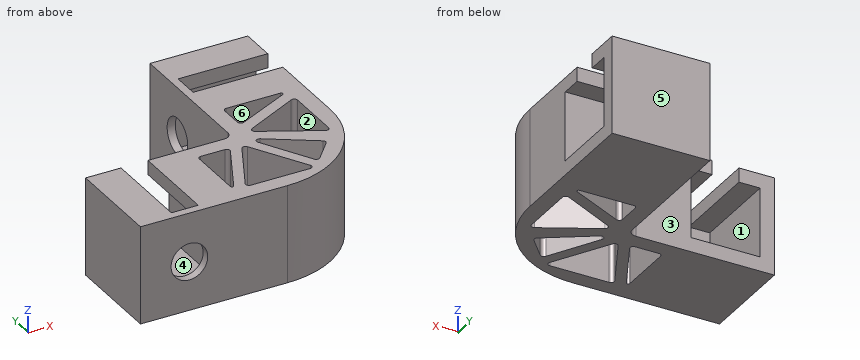
Autodesk Inventor part; units mm, degrees
ref_plane "YZ Plane" through (0, 0, 0) normal (1, 0, 0) x (0, 1, 0)
ref_plane "XZ Plane" through (0, 0, 0) normal (0, 1, 0) x (-1, 0, 0)
ref_plane "XY Plane" through (0, 0, 0) normal (0, 0, 1) x (1, 0, 0)
sketch "Sketch1" plane through (0, 0, 0) normal (0, 0, 1) x (1, 0, 0)
  line L0 (0, 0) -> (150, 0)
  line L1 (150, 0) -> (150, 45)
  line L2 (90, 60) -> (0, 60)
  line L3 (0, 60) -> (0, 0)
  line L4 (90, 60) -> (90, 150)
  line L5 (90, 150) -> (150, 150)
  line L6 (150, 150) -> (150, 45)
  dimension "d5" = 90
  dimension "d6" = 60
  dimension "d7" = 90
  dimension "d9" = 60
  dimension "d10" = 150
  dimension "d11" = 150
extrude "Extrusion1" add sketch "Sketch1" along normal blind 60
sketch "Sketch2" plane through (0, 60, 0) normal (0, 1, 0) x (1, 0, 0)
  line L0 (0, 0) -> (150, 0) construction
  line L1 (0, 0) -> (60, -60) construction
  line L2 (0, 0) -> (84.8528, 0) construction
  line L3 (8.75, -51.25) -> (8.75, -8.75)
  line L4 (8.75, -8.75) -> (51.25, -8.75)
  line L5 (51.25, -8.75) -> (51.25, -51.25)
  line L6 (51.25, -51.25) -> (8.75, -8.75) construction
  line L7 (8.75, -51.25) -> (51.25, -8.75) construction
  line L8 (30, -30) -> (30, -51.25) construction
  line L9 (30, -51.25) -> (21.75, -51.25) construction
  line L10 (30, -51.25) -> (38.25, -51.25) construction
  line L11 (21.75, -51.25) -> (21.75, -60)
  line L12 (0, -60) -> (150, -60)
  line L13 (38.25, -51.25) -> (38.25, -60)
  line L14 (21.75, -60) -> (38.25, -60)
  line L15 (51.25, -51.25) -> (38.25, -51.25)
  line L16 (21.75, -51.25) -> (8.75, -51.25)
  dimension "d14" = 84.8528
  dimension "d15" = 45
  dimension "d16" = 42.5
  dimension "d17" = 42.5
  dimension "d32" = 8.25
  dimension "d33" = 8.25
  dimension "d34" = 90
extrude "Extrusion2" cut sketch "Sketch2" against normal blind 55
sketch "Sketch4" plane through (150, 0, 0) normal (1, 0, 0) x (0, 0, -1)
  line L0 (0, 150) -> (0, 60) construction
  line L1 (0, 150) -> (-60, 90) construction
  line L2 (0, 150) -> (84.8528, 150) construction
  line L3 (-51.25, 98.75) -> (-8.75, 98.75)
  line L4 (-8.75, 98.75) -> (-8.75, 141.25)
  line L5 (-8.75, 141.25) -> (-51.25, 141.25)
  line L6 (-51.25, 98.75) -> (-8.75, 141.25) construction
  line L7 (-8.75, 98.75) -> (-51.25, 141.25) construction
  line L8 (-30, 120) -> (-60, 120) construction
  line L9 (-60, 120) -> (-60, 128.25)
  line L10 (-60, 0) -> (-60, 150)
  line L11 (-60, 128.25) -> (-51.25, 128.25)
  line L12 (-60, 120) -> (-60, 111.75)
  line L13 (-60, 111.75) -> (-51.25, 111.75)
  line L14 (-51.25, 141.25) -> (-51.25, 128.25)
  line L15 (-51.25, 111.75) -> (-51.25, 98.75)
  point P0 (0, 0)
  dimension "d26" = 84.8528
  dimension "d27" = 135
  dimension "d28" = 42.5
  dimension "d29" = 42.5
  dimension "d35" = 8.25
  dimension "d36" = 8.25
  dimension "d37" = 90
extrude "Extrusion4" cut sketch "Sketch4" against normal blind 55
hole "Hole2" at (30, 5, 30) direction (0, -1, 0) diameter 22.5 end through all
hole "Hole4" at (95, 120, 30) direction (-1, 0, 0) diameter 22.5 end through all
fillet "Fillet1" radius 5 1 edges at (90, 60, 30)
fillet "Fillet2" radius 60 1 edges at (150, 0, 30)
sketch "Sketch5" plane through (0, 0, 60) normal (0, 0, 1) x (1, 0, 0)
  line L0 (0, 0) -> (90, 0) construction
  line L1 (0, 0) -> (60, 0) construction
  line L2 (60, 0) -> (60, 60) construction
  line L3 (60, 60) -> (0, 60) construction
  line L4 (0, 60) -> (0, 0) construction
  line L5 (149.6513, 150.4559) -> (89.6513, 150.4559) construction
  line L6 (89.6513, 150.4559) -> (89.6513, 90.4559) construction
  line L7 (89.6513, 90.4559) -> (149.6513, 90.4559) construction
  line L8 (149.6513, 90.4559) -> (149.6513, 150.4559) construction
  line L9 (89.6513, 90.4559) -> (149.6513, 90.4559) construction
  line L10 (149.6513, 90.4559) -> (149.6513, 80.4559) construction
  line L11 (149.6513, 80.4559) -> (89.6513, 80.4559) construction
  line L12 (89.6513, 80.4559) -> (89.6513, 90.4559) construction
  line L13 (60, 60) -> (70, 60) construction
  line L14 (70, 60) -> (70, 0) construction
  line L15 (70, 0) -> (60, 0) construction
  line L16 (60, 0) -> (60, 60) construction
  line L17 (70, 60) -> (89.6513, 60) construction
  line L18 (89.6513, 60) -> (89.6513, 80.4559) construction
  line L19 (89.6513, 80.4559) -> (70, 80.4559) construction
  line L20 (70, 80.4559) -> (70, 60) construction
  line L21 (70, 60) -> (90, 60) construction
  line L22 (90, 60) -> (90, 50) construction
  line L23 (90, 50) -> (70, 50) construction
  line L24 (70, 50) -> (70, 60) construction
  line L25 (90, 50) -> (100, 50) construction
  line L26 (100, 50) -> (100, 60.8297) construction
  line L27 (100, 60.8297) -> (90, 60.8297) construction
  line L28 (90, 60.8297) -> (90, 50) construction
  line L29 (100, 60.8297) -> (89.6513, 60.8297) construction
  line L30 (89.6513, 60.8297) -> (89.6513, 80.4559) construction
  line L31 (89.6513, 80.4559) -> (100, 80.4559) construction
  line L32 (100, 80.4559) -> (100, 60.8297) construction
  line L33 (149.6513, 80.4559) -> (139.6513, 80.4559) construction
  line L34 (139.6513, 80.4559) -> (139.6513, 0.4559) construction
  line L35 (139.6513, 0.4559) -> (149.6513, 0.4559) construction
  line L36 (149.6513, 0.4559) -> (149.6513, 80.4559) construction
  line L37 (70, 0) -> (139.6513, 0) construction
  line L38 (139.6513, 0) -> (139.6513, 10) construction
  line L39 (139.6513, 10) -> (70, 10) construction
  line L40 (70, 10) -> (70, 0) construction
  arc A0 (90, 0) -> (150, 60) centre (90, 60) ccw construction
  line L41 (123.1662, 10) -> (113.1662, 10) construction
  line L42 (113.1662, 10) -> (113.1662, 20) construction
  line L43 (113.1662, 20) -> (123.1662, 20) construction
  line L44 (123.1662, 20) -> (123.1662, 10) construction
  line L45 (123.1662, 20) -> (133.1662, 20) construction
  line L46 (133.1662, 20) -> (133.1662, 30) construction
  line L47 (133.1662, 30) -> (123.1662, 30) construction
  line L48 (123.1662, 30) -> (123.1662, 20) construction
  line L49 (133.1662, 30) -> (143.1662, 30) construction
  line L50 (143.1662, 30) -> (143.1662, 40) construction
  line L51 (143.1662, 40) -> (133.1662, 40) construction
  line L52 (133.1662, 40) -> (133.1662, 30) construction
  line L53 (70, 10) -> (90, 50)
  line L54 (113.1662, 10) -> (90, 50)
  line L55 (70, 10) -> (113.1662, 10)
  line L56 (100, 60.8297) -> (139.6513, 40)
  line L57 (100, 60.8297) -> (139.6513, 80.4559)
  line L58 (139.6513, 40) -> (139.6513, 80.4559)
  line L59 (113.1662, 10) -> (139.6513, 40) construction
  line L60 (90, 50) -> (100, 60.8297) construction
  line L61 (95, 55.4149) -> (117.8355, 15.289)
  line L62 (95, 55.4149) -> (131.9763, 31.3064)
  line L63 (117.8355, 15.289) -> (131.9763, 31.3064)
  line L64 (90, 50) -> (83, 50) construction
  line L65 (83, 50) -> (63.0073, 10)
  line L66 (63.0073, 10) -> (63.0073, 50)
  line L67 (63.0073, 50) -> (83, 50)
  line L68 (100, 69.1023) -> (139.6513, 88.1548)
  line L69 (139.6513, 88.1548) -> (100, 88.1548)
  line L70 (100, 88.1548) -> (100, 69.1023)
  dimension "d76" = 60
  dimension "d77" = 60
  dimension "d78" = 60
  dimension "d79" = 60
  dimension "d80" = 60
  dimension "d81" = 10
  dimension "d82" = 10
  dimension "d83" = 60
  dimension "d84" = 10
  dimension "d85" = 10
  dimension "d86" = 10
  dimension "d87" = 80
  dimension "d88" = 10
  dimension "d89" = 10
  dimension "d90" = 10
  dimension "d91" = 10
  dimension "d92" = 10
  dimension "d93" = 10
  dimension "d94" = 10
  dimension "d97" = 7
extrude "Extrusion5" cut sketch "Sketch5" against normal blind 94
fillet "Fillet3" radius 2 13 edges at (113.1662, 10, 30) (131.9763, 31.3064, 30) (117.8355, 15.289, 30) (70, 10, 30) (63.0073, 50, 30) (83, 50, 30) (90, 50, 30) (95, 55.4149, 30) (100, 60.8297, 30) (100, 69.1023, 30) (100, 88.1548, 30) (139.6513, 80.4559, 30) (139.6513, 40, 30)
fillet "Fillet4" radius 1 2 edges at (63.0073, 10, 30) (139.6513, 88.1548, 30)
properties part number "OuterFrame"
The listing builds one solid part. Answer for the finished solid, in the listing's coordinates (mm). Face numbers are marked on the shaded views. A direction names the side the tool comes from. Give positions to 0.01 mm unless a question says otherwise; leave off trailing zeros. Order: outer loops, then holes, each group sorted by start corner. A loop starts at its lowest first (then second) coordinate and runs counter-clockwise, first axis right, second up. Notation, with made-up numbers: (-13.5, 34) -> (39.5, 34) arc R28 ccw to (39.5, 62) -> close; hole circle Ø11 at (83, 85). An arc over 180 degrees is marked (long way). Answer as CSV lines item,"result". Start each with the question number.
Q1. A cutting plane is placed at B-B (y = 120). Determine the outline of the cut face in (x, z).
Q2. Which of the six approach directions +Z, -Z, +X, -X, +Y, -Y give full straight-line access (tool end or side, diameter ignored) to the marked faces 1, 2 and 3?
Q3. Given pin 1 (5 mm diameter, centred on y = 31.5, z = 30, fed in from +X); pin 2 (3 mm diameter, centred on x = 35, y = 30, fed in from +Z); pin 3 (2 mm diameter, centred on y = 34.5, z = 7, fed in from +X), each flat-ended and moving along its own axis, determine where each tip first touches the part or whether it passes through.
Q4. A cutting plane is placed at C-C (z = 21). Count the separate pieces of the cut face and the enclosed holes in it, then the cut area to 3 significant figures.
Q5. A cutting plane is placed at D-D (y = 101). Determine the outline of the cut face in (x, z), then the cut area to 3 significant figures.
Q6. A cutting plane is placed at A-A (x = 30). Determine the outline of the cut face in (y, z), then the cut area to 3 significant figures.
Q7. Find the intervals of material crossed by L1, parallel to X at y = 72.5, z = 30.5; L2, parallel to Y at x = 93.5, z = 30; L3, parallel to Y at x = 101.5, z = 33, in increasing order.
Q8. Determine the mould class of the marked faces 4, 5 and 6 for opening direction Y: pulls with the +Y half, pulls with the -Y half, needs draft (parallel to the pull), parting line crosses it, or undercut.
Results found:
1,outline,"(90, 0) -> (150, 0) -> (150, 8.75) -> (95, 8.75) -> (95, 18.75) -> (90, 18.75) -> close; (90, 41.25) -> (95, 41.25) -> (95, 60) -> (90, 60) -> close"
2,face 1,"+Y"
2,face 2,"+Z, -Z"
2,face 3,"+Z, -Z, -X, +Y"
3,pin 1,"x = 144.07"
3,pin 2,"z = 8.75"
3,pin 3,"x = 144.77"
4,separate pieces,"3"
4,enclosed holes,"5"
4,area,"5,960 mm2"
5,outline,"(90, 0) -> (150, 0) -> (150, 8.75) -> (95, 8.75) -> (95, 51.25) -> (150, 51.25) -> (150, 60) -> (90, 60) -> close"
5,area,"1,260 mm2"
6,outline,"(0, 0) -> (60, 0) -> (60, 8.75) -> (5, 8.75) -> (5, 18.75) -> (0, 18.75) -> close; (0, 41.25) -> (5, 41.25) -> (5, 60) -> (0, 60) -> close"
6,area,"669 mm2"
7,L1,"90 to 100, 107.07 to 123.58, 139.65 to 150"
7,L2,"0.1 to 10, 43.96 to 108.75, 131.25 to 150"
7,L3,"1.11 to 10, 30.14 to 43.99, 51.11 to 70.35, 88.09 to 98.75, 141.25 to 150"
8,face 4,"needs draft"
8,face 5,"pulls with the +Y half"
8,face 6,"undercut"
